The listing builds one solid part. Answer for the finished solid, in the listing's coordinates (mm). A direction names the side the tool comes from. Round coordinates to 2 decimals unless told otherwise and drop trailing zeros. Loops run counter-clockwise (first coordinate to the right, second up) from the corner with the lowest first, then second, coordinate; pieces in that order, holes last. Notation, with made-up numbers: (-2.75, 19.5) -> (6.25, 19.5) arc R25 ccw to (6.25, 45.5) -> close; hole circle Ø11 at (39, 9). An arc over 180 degrees is marked (long way). Write each question's results on one line, items separated by ' | '. Start each with the question number.
(1) The part is cut by section C-C (z = -9). Determine the outline of the cut face in (x, y).
(2) Straight lines are drawn through the part: probe 1 along Y at (x, z) = (5.5, -6.75); probe 2 along Z at (x, y) = (-49, -3); probe 3 along Y at (x, z) = (12.5, -1.5). For each, find the intervals that lie inside material, in ascending order.
(3) The part is cut by section D-D (x = -57). Determine the outline of the cut face in (y, z).
(4) The part is cut by section B-B (y = 22.5). Determine the outline of the cut face in (x, z).
(5) Determine the mould class of faces 6 (the face through (8, 9, -3)), 7 (the face through (6, 9, -5.75)), 8 (the face through (9.9, 0.5, -16.5)), 9 (the face through (-7.36, 15.9, -3.82)) for opening direction Y: released by +Y, released by -Y, zero draft, split by the parting line, or undercut.
(6) Flat-ended cylindrical pins translate along their axes: pin 1 (3 mm diameter, centred on y = 9.5, z = -12, fed in from -X); pin 2 (4 mm diameter, centred on y = 12, z = -15.5, fed in from +X); pin 3 (1.5 mm diameter, centred on y = -3, z = -6, fed in from +X) (3 decimals). Find the tip coordinate at first contact, or state that the pin passes through.
(7) For faces 1 (the face through (0, 9, -15)), 2 (the face through (0, 22, -2)), 3 (the face through (12, 1, -7.2)), 4 (the face through (12, -2, -10)), 5 (the face through (8, 9, -18)), determine the directions among +Z, -Z, +X, -X, +Y, -Y from which every point of the face is accessible in a straight line to the end or side of a thin tool.
```python
from build123d import *

# Parameters (mm, degrees)
SKETCH_1_W          = 10
SKETCH_1_H          = 19
EXTRUDE_1_DEPTH     = 6.5
EXTRUDE_2_DEPTH     = 7
FILLET_1_R          = 3
SKETCH_3_W          = 5
SKETCH_3_H          = 30
EXTRUDE_3_DEPTH     = 8
SKETCH_4_W          = 8
SKETCH_4_H          = 19
EXTRUDE_4_DEPTH     = 15
SKETCH_6_W          = 11
SKETCH_6_H          = 13
CUT_EXTRUDE_1_DEPTH = 4
SKETCH_8_W          = 9.1
SKETCH_8_H          = 20
EXTRUDE_5_DEPTH     = 3
SKETCH_8_2_W        = 9.1
SKETCH_8_2_H        = 20
EXTRUDE_6_DEPTH     = 2
FILLET_2_R          = 3.5
FILLET_3_R          = 3


with BuildPart() as part:
    # 草圖1 → 填料-伸長1 (new body)
    with BuildSketch(Plane(origin=(0, 0, 0), x_dir=(0, 0, -1), z_dir=(1, 0, 0))):
        with Locations((5, 9.5)):
            Rectangle(SKETCH_1_W, SKETCH_1_H)
    extrude(amount=-EXTRUDE_1_DEPTH)

    # 草圖2 → 填料-伸長2 (add)
    with BuildSketch(Plane.XY):
        with BuildLine():
            Line((-11.419601085, 15), (-6.5, 15))
            Line((-6.5, 15), (-6.5, 4))
            Line((-6.5, 4), (-11.606123087, 4))
            ThreePointArc((-11.606123087, 4), (-70.995688063, 10.508623254), (-11.419601085, 15))
        make_face()
    extrude(amount=-EXTRUDE_2_DEPTH)

    # 圓角1
    fillet_1_edges = [part.edges().sort_by_distance(p)[0] for p in [
        (-6.5, 9.5, -7),
    ]]
    fillet(fillet_1_edges, radius=FILLET_1_R - 0.0001)  # a hair under: the kernel refuses the full size

    # 草圖3 → 填料-伸長3 (add)
    with BuildSketch(Plane(origin=(0, 0, 0), x_dir=(0, 0, -1), z_dir=(1, 0, 0))):
        with Locations((2.5, 9.5)):
            Rectangle(SKETCH_3_W, SKETCH_3_H)
    extrude(amount=EXTRUDE_3_DEPTH)

    # 草圖4 → 填料-伸長4 (add)
    with BuildSketch(Plane(origin=(0, 0, -5), x_dir=(-1, 0, 0), z_dir=(0, 0, -1))):
        with Locations((-4, 9.5)):
            Rectangle(SKETCH_4_W, SKETCH_4_H)
    extrude(amount=EXTRUDE_4_DEPTH)

    # 草圖6 → 除料-伸長1 (cut)
    with BuildSketch(Plane(origin=(8, 0, 0), x_dir=(0, 0, -1), z_dir=(1, 0, 0))):
        with Locations((11.25, 9.5)):
            Rectangle(SKETCH_6_W, SKETCH_6_H)
    extrude(amount=-CUT_EXTRUDE_1_DEPTH, mode=Mode.SUBTRACT)

    # 草圖8 → 填料-伸長5 (add)
    with BuildSketch(Plane(origin=(0, 19, 0), x_dir=(1, 0, 0), z_dir=(0, 1, 0))):
        with Locations((12.55, 10)):
            Rectangle(SKETCH_8_W, SKETCH_8_H)
        with BuildLine():
            Line((13.6, 15.3), (11.1, 15.3))
            ThreePointArc((11.1, 15.3), (9.9, 16.5), (11.1, 17.7))
            Line((11.1, 17.7), (13.6, 17.7))
            ThreePointArc((13.6, 17.7), (14.8, 16.5), (13.6, 15.3))
        make_face(mode=Mode.SUBTRACT)
        with BuildLine():
            Line((13.6, 4.8), (11.1, 4.8))
            ThreePointArc((11.1, 4.8), (9.9, 6), (11.1, 7.2))
            Line((11.1, 7.2), (13.6, 7.2))
            ThreePointArc((13.6, 7.2), (14.8, 6), (13.6, 4.8))
        make_face(mode=Mode.SUBTRACT)
    extrude_5 = extrude(amount=-EXTRUDE_5_DEPTH)

    # 鏡射1: 填料-伸長5 across plane
    add(extrude_5.mirror(Plane.ZX.offset(9.5)))

    # 草圖8<2> → 填料-伸長6 (add)
    with BuildSketch(Plane(origin=(0, 19, 0), x_dir=(1, 0, 0), z_dir=(0, 1, 0))):
        with Locations((12.55, 10)):
            Rectangle(SKETCH_8_2_W, SKETCH_8_2_H)
        with BuildLine():
            Line((13.6, 15.3), (11.1, 15.3))
            ThreePointArc((11.1, 15.3), (9.9, 16.5), (11.1, 17.7))
            Line((11.1, 17.7), (13.6, 17.7))
            ThreePointArc((13.6, 17.7), (14.8, 16.5), (13.6, 15.3))
        make_face(mode=Mode.SUBTRACT)
        with BuildLine():
            Line((13.6, 4.8), (11.1, 4.8))
            ThreePointArc((11.1, 4.8), (9.9, 6), (11.1, 7.2))
            Line((11.1, 7.2), (13.6, 7.2))
            ThreePointArc((13.6, 7.2), (14.8, 6), (13.6, 4.8))
        make_face(mode=Mode.SUBTRACT)
    extrude_6 = extrude(amount=EXTRUDE_6_DEPTH)

    # 鏡射2: 填料-伸長6 across plane
    add(extrude_6.mirror(Plane.ZX.offset(9.5)))

    # 圓角2
    fillet_2_edges = [part.edges().sort_by_distance(p)[0] for p in [
        (8, 24.5, -2.5),
        (8, -5.5, -2.5),
    ]]
    fillet(fillet_2_edges, radius=FILLET_2_R - 0.0001)  # a hair under: the kernel refuses the full size

    # 圓角3
    fillet_3_edges = [part.edges().sort_by_distance(p)[0] for p in [
        (-6.5, 4, -4.99995),
        (-6.5, 15, -4.99995),
    ]]
    fillet(fillet_3_edges, radius=FILLET_3_R - 0.0001)  # a hair under: the kernel refuses the full size


solid = part.part
```
Checked values:
1) outline: (-6.67, 2) arc R3 cw to (-6.5, 1) -> (-6.5, 0) -> (8, 0) -> (8, -2) -> (17.1, -2) -> (17.1, 3) -> (4, 3) -> (4, 16) -> (17.1, 16) -> (17.1, 21) -> (8, 21) -> (8, 19) -> (-6.5, 19) -> (-6.5, 18) arc R3 cw to (-6.67, 17) -> close
2) probe 1: y = 0 to 3, 16 to 19 | probe 2: z = -7 to 0 | probe 3: y = -2 to 3, 16 to 21
3) outline: (-15.38, -7) -> (35.38, -7) -> (35.38, 0) -> (-15.38, 0) -> close
4) outline: (-68.27, -7) -> (-13.73, -7) -> (-13.73, 0) -> (-68.27, 0) -> close; (0, -5) -> (7.66, -5) -> (7.66, 0) -> (0, 0) -> close
5) face 6: undercut | face 7: undercut | face 8: zero draft | face 9: released by +Y
6) pin 1: stops at x = 0 | pin 2: stops at x = 8 | pin 3: stops at x = -13.615
7) face 1: -Z, -X, +Y, -Y | face 2: +Z, -Z, +Y | face 3: +Y, -Y | face 4: +Z, -Z, +X, -Y | face 5: +Z, -Z, +X
